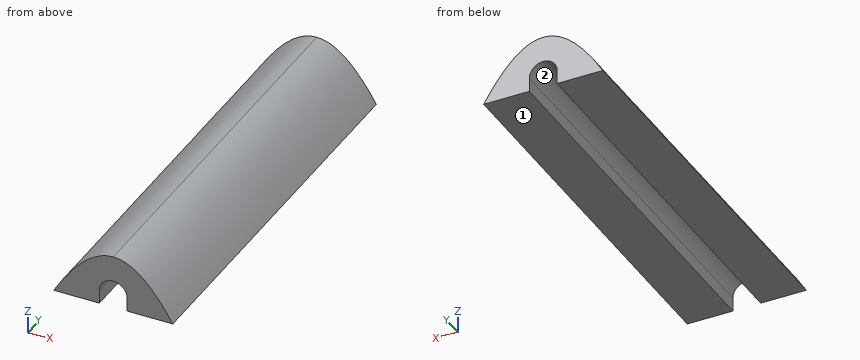
Autodesk Fusion 360 part; units mm, degrees
sketch "Sketch1" plane through (0, 0, 0) normal (0, 1, 0) x (1, 0, 0)
  line L0 (0, 0) -> (6, 0)
  line L1 (3, 0) -> (3, -0.7)
  circle A0 centre (3, -0.7) radius 0.7
  line L2 (3, -0.7) -> (3, -2.7)
  spline S0 degree 5 poles (0, 0) (0.12, -0.2048) (0.36, -0.5965) (0.72, -1.1304) (1.2, -1.7331) (1.8, -2.2925) (2.4, -2.6403) (3, -2.7594) (3.6, -2.6403) (4.2, -2.2925) (4.8, -1.7331) (5.28, -1.1304) (5.64, -0.5965) (5.88, -0.2048) (6, 0) knots 0 0 0 0 0 0 0.1 0.2 0.3 0.4 0.5 0.6 0.7 0.8 0.9 1 1 1 1 1 1
  line L3 (3, -0.7) -> (2.3, -0.7)
  line L4 (2.3, -0.7) -> (2.3, 0)
  line L5 (3, -0.7) -> (3.7, -0.7)
  line L6 (3.7, -0.7) -> (3.7, 0)
  dimension "d1" = 6
  dimension "d2" = 0.7
  dimension "d3" = 2
extrude "Extrude1" add sketch "Sketch1" along normal blind 20 contours L0 A0 L2 S0 L4 | L0 A0 L2 S0 L6
Model file for the job. Use its own axes, mm. Face numbers are marked on the shaded views. Coordinates: 2 decimals unless noted, no trailing zeros. Return JSON: item names as keys, results as strings.
1. Drill centre lines: probe 1 along X at (y, z) = (8.75, 1.15); probe 2 along Z at (x, y) = (3, 1.5); probe 3 along X at (y, z) = (14.25, 0.75). Where is each one in solid material? Low to high.
Ans:
{"probe 1": "0.76 to 2.46, 3.54 to 5.24", "probe 2": "1.4 to 2.7", "probe 3": "0.47 to 2.3, 3.7 to 5.53"}
2. Flat gauge pin, fed straight in: pin 1 (1 mm diameter, centred on y = 13.5, z = 1.5, fed in from +X). Where does the tip first touch, or does it go through?
Ans:
{"pin 1": "x = 5.35"}
3. Pull direction X, two halves, no side cores. Call the marked faces 1 and 2: +X half, -X half, draft (parallel to the pull), parting line (faces both ways), or undercut.
Ans:
{"face 1": "draft", "face 2": "undercut"}
